```python
from build123d import *

# Parameters (mm, degrees)
BOSS_EXTRUDE1_DEPTH = 21
SKETCH2_W           = 42
SKETCH2_H           = 72
BOSS_EXTRUDE2_DEPTH = 10
BOSS_EXTRUDE3_DEPTH = 35
CHAMFER1_SIZE       = 20
FILLET1_R           = 1


with BuildPart() as part:
    # Sketch1 → Boss-Extrude1 (new, symmetric)
    with BuildSketch(Plane(origin=(0, 0, 0), x_dir=(0, 0, -1), z_dir=(1, 0, 0))):
        Polygon((0, -9.2), (0, 9.2), (40, 9.2), (40, 19.2), (-10, 19.2), (-10, -19.2), (40, -19.2), (40, -9.2), align=None)
    extrude(amount=BOSS_EXTRUDE1_DEPTH, both=True)

    # Sketch2 → Boss-Extrude2 (add)
    with BuildSketch(Plane.XY.offset(10)):
        Rectangle(SKETCH2_W, SKETCH2_H)
    extrude(amount=BOSS_EXTRUDE2_DEPTH)

    # Sketch3 → Boss-Extrude3 (add)
    with BuildSketch(Plane.XY.offset(20)):
        Polygon((-15.2, 30.2), (-15.2, 24), (-21, 24), (-21, 36), (21, 36), (21, 24), (15.2, 24), (15.2, 30.2), align=None)
        Polygon((-15.2, -30.2), (15.2, -30.2), (15.2, -24), (21, -24), (21, -36), (-21, -36), (-21, -24), (-15.2, -24), align=None)
    extrude(amount=BOSS_EXTRUDE3_DEPTH)

    # Chamfer1
    # the kernel refuses this chamfer: 20 mm, written as the material it adds along each edge
    with BuildSketch(Plane(origin=(-21, -19.2, 10), x_dir=(0, 0.027495876610586317, -0.9996219169112968), z_dir=(1, 0, 0))) as chamfer1_piece_1_section:
        Polygon((CHAMFER1_SIZE * 0.999621916911, -CHAMFER1_SIZE * 0.0274958766106), (-CHAMFER1_SIZE * 0.0274958766106, -CHAMFER1_SIZE * 0.999621916911), (0, 0), align=None)
    chamfer1_piece_1 = extrude(amount=42, mode=Mode.PRIVATE)
    chamfer1_piece_1 = split(chamfer1_piece_1, bisect_by=Plane(origin=(0, -36, 3.17327651), z_dir=(0, 1, 0)), keep=Keep.TOP, mode=Mode.PRIVATE)
    add(chamfer1_piece_1)
    with BuildSketch(Plane(origin=(-21, 19.2, 10), x_dir=(0, 0.9996219169112968, 0.027495876610586403), z_dir=(1, 0, 0))) as chamfer1_piece_2_section:
        Polygon((CHAMFER1_SIZE * 0.999621916911, -CHAMFER1_SIZE * 0.0274958766106), (-CHAMFER1_SIZE * 0.0274958766106, -CHAMFER1_SIZE * 0.999621916911), (0, 0), align=None)
    chamfer1_piece_2 = extrude(amount=42, mode=Mode.PRIVATE)
    chamfer1_piece_2 = split(chamfer1_piece_2, bisect_by=Plane(origin=(0, 36, 3.17327651), z_dir=(0, -1, 0)), keep=Keep.TOP, mode=Mode.PRIVATE)
    add(chamfer1_piece_2)

    # Fillet1
    fillet1_edges = [part.edges().sort_by_distance(p)[0] for p in [
        (-21, 19.2, -25),
        (-21, 14.2, -40),
        (21, -14.2, -40),
        (21, -9.2, -20),
        (-21, 36, 30.9),
        (-21, -36, 30.9),
        (21, -36, 30.9),
        (21, 36, 30.9),
        (21, 0, 0),
        (21, 9.2, -20),
        (-21, 0, 20),
        (21, 24, 37.5),
        (-21, 24, 37.5),
        (0, 30.2, 55),
        (15.2, 27.1, 55),
        (18.1, 24, 55),
        (21, 30, 55),
        (0, 36, 55),
        (-21, 30, 55),
        (-18.1, 24, 55),
        (-15.2, 27.1, 55),
        (21, 14.2, -40),
        (21, 0, 20),
        (-21, -24, 37.5),
        (21, -24, 37.5),
        (-15.2, -27.1, 55),
        (-18.1, -24, 55),
        (-21, -30, 55),
        (0, -36, 55),
        (21, -30, 55),
        (18.1, -24, 55),
        (15.2, -27.1, 55),
        (0, -30.2, 55),
        (-21, -19.2, -25),
        (21, -19.2, -25),
        (-21, -27.6, -1.6),
        (0, -36, 6.8),
        (21, -27.6, -1.6),
        (-21, 9.2, -20),
        (0, 36, 6.8),
        (-21, 27.6, -1.6),
        (21, 27.6, -1.6),
        (21, 19.2, -25),
        (-21, 0, 0),
        (-21, -9.2, -20),
        (-21, -14.2, -40),
    ]]
    fillet(fillet1_edges, radius=FILLET1_R)


solid = part.part
```
Geometry: final body of the model. Coordinates: model frame, mm. A direction names the side the tool comes from. Coordinates: 2 decimals unless noted, no trailing zeros. Loops run counter-clockwise (first coordinate to the right, second up) from the corner with the lowest first, then second, coordinate; pieces in that order, holes last. Notation, with made-up numbers: M 69,11.5 L 74,11.5 A23 cw 74,37.5 Z; hole C 46,68 d1. An arc over 180 degrees is marked long. Put each result on its own line as item: value.
(1) Cut plane A-A on z = 31. Return the cut outline in (x, y), then the cut area to 3 significant figures.
Answer sheet:
outline: M -21,-35 A1 ccw -20,-36 L 20,-36 A1 ccw 21,-35 L 21,-25 A1 ccw 20,-24 L 15.2,-24 L 15.2,-30.2 L -15.2,-30.2 L -15.2,-24 L -20,-24 A1 ccw -21,-25 Z; M -21,25 A1 ccw -20,24 L -15.2,24 L -15.2,30.2 L 15.2,30.2 L 15.2,24 L 20,24 A1 ccw 21,25 L 21,35 A1 ccw 20,36 L -20,36 A1 ccw -21,35 Z
area: 629 mm^2
(2) Material intervals for probe 1 along Y at (x, z) = (-9.5, 23.5); probe 2 along Y at (x, z) = (16, 30.5); probe 3 along X at (y, z) = (-26, 40), sorted ascending.
Answer sheet:
probe 1: y = -36 to -30.2, 30.2 to 36
probe 2: y = -36 to -24, 24 to 36
probe 3: x = -21 to -15.2, 15.2 to 21
(3) Access query for faces 1 (the face through (0, -9.2, -20)), 2 (the face through (0, 19.2, -25)), 3 (the face through (-18, -24, 37)), 4 (the face through (15.2, 27, 37)). Directions: +Z, -Z, +X, -X, +Y, -Y. A direction counts if a zero-diameter tool reaches every point of the face in a straight line with its end or side. Return the directions, or none.
Answer sheet:
face 1: -Z, +X, -X
face 2: -Z, +X, -X, +Y
face 3: +Z, +X, -X
face 4: +Z
(4) Draft query along X for faces 5 (the face through (-15.2, 27, 37)), 6 (the face through (0, -32, 55)), 7 (the face through (-20.699, -27.223, -1.574)). Return one class per face: pulls with the +X half, pulls with the -X half, needs draft (parallel to the pull), parting line crosses it, or undercut.
Answer sheet:
face 5: undercut
face 6: needs draft
face 7: pulls with the -X half
(5) Cut plane D-D on z = -26. Return the cut outline in (x, y), then the cut area to 3 significant figures.
Answer sheet:
outline: M -21,-18.2 A1 ccw -20,-19.2 L 20,-19.2 A1 ccw 21,-18.2 L 21,-10.2 A1 ccw 20,-9.2 L -20,-9.2 A1 ccw -21,-10.2 Z; M -21,10.2 A1 ccw -20,9.2 L 20,9.2 A1 ccw 21,10.2 L 21,18.2 A1 ccw 20,19.2 L -20,19.2 A1 ccw -21,18.2 Z
area: 838 mm^2
(6) First-contact query: pin 1 (8 mm diameter, centred on x = -5, z = -22, fed in from -Y); pin 2 (5 mm diameter, centred on x = 15, y = 5.5, fed in from -Z); pin 3 (1.5 mm diameter, centred on x = -9, y = 22, fed in from +Z). Flat tips, straight axial feed; report the tip coordinate or a pass-through.
Answer sheet:
pin 1: stops at y = -19.2
pin 2: stops at z = 0
pin 3: stops at z = 20
(7) Cut plane B-B on x = 2. Return the cut outline in (y, z).
Answer sheet:
outline: M -36,7.21 A1 ccw -35.71,6.51 L -19.2,-10 L -19.2,-40 L -9.2,-40 L -9.2,0 L 9.2,0 L 9.2,-40 L 19.2,-40 L 19.2,-10 L 35.71,6.51 A1 ccw 36,7.21 L 36,54 A1 ccw 35,55 L 31.2,55 A1 ccw 30.2,54 L 30.2,20 L -30.2,20 L -30.2,54 A1 ccw -31.2,55 L -35,55 A1 ccw -36,54 Z
(8) Cut plane C-C on y = -6. Return the cut outline in (x, z), then the cut area to 3 significant figures.
Answer sheet:
outline: M -21,1 A1 ccw -20,0 L 20,0 A1 ccw 21,1 L 21,19 A1 ccw 20,20 L -20,20 A1 ccw -21,19 Z
area: 839 mm^2
